```python
from build123d import *

# Parameters (mm, degrees)
F2_R      = 40
F2_R_2    = 23
F4_DEPTH  = 34
F8_DEPTH  = 25
F10_DEPTH = 34


with BuildPart() as f4:
    # F2 (on face) → F4 (new body)
    with BuildSketch(Plane(origin=(0, 0, 0), x_dir=(-1, 0, 0), z_dir=(0, 0.906308, 0.422618))):
        Circle(F2_R)
        Circle(F2_R_2, mode=Mode.SUBTRACT)
    extrude(amount=-F4_DEPTH)



with BuildPart() as f8:
    # F7 (on offset) → F8 (new body)
    with BuildSketch(Plane.YZ.offset(-46)):
        Polygon((-14.199466, -50), (-33.909734, -50), (-33.909734, -65), (-13.909734, -65), (-13.909734, -50.621332), align=None)
        Polygon((-13.909734, -50.621332), (-13.909734, -65), (-7.204851, -65), align=None)
        Polygon((23.315383, -50), (-14.199466, -50), (-13.909734, -50.621332), (-7.204851, -65), (30.309998, -65), align=None)
        Polygon((46.090266, -50), (23.315383, -50), (30.309998, -65), (46.090266, -65), align=None)
    extrude(amount=F8_DEPTH)


with BuildPart() as f4_1:
    add(f4.part)

    add(f8.part)  # F10 merges F8
    # F9 (on face) → F10 (join, through all)
    with BuildSketch(Plane(origin=(0, 0, 0), x_dir=(-1, 0, 0), z_dir=(0, 0.906308, 0.422618))):
        with BuildLine():
            Line((40, -85.627586), (40, 0))
            ThreePointArc((40, 0), (35.496479, -18.439089), (23, -32.726136))
            Line((23, -32.726136), (23, -85.627586))
            Line((23, -85.627586), (40, -85.627586))
        make_face()
    extrude(amount=-F10_DEPTH)


solid = f4_1.part
```
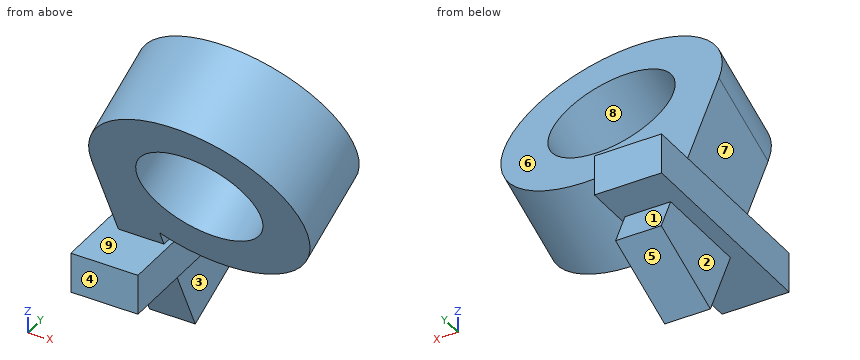
CAD build for the part. Positions are in the model's coordinates, mm. Face numbers are marked on the shaded views. A direction names the side the tool comes from. Round coordinates to 2 decimals unless told otherwise and drop trailing zeros. Write each loop counter-clockwise with the first axis right and the second up, starting at its lowest first coordinate (ties: lowest second). Pieces come first, ordered by that corner, then holes.
Item 1: Drill centre lines: L1, parallel to Z at x = -22.5, y = 5; L2, parallel to Z at x = 0, y = -16; L3, parallel to X at y = -2.5, z = -65.5. Where is each one in solid material? Low to high.
Filled in:
L1: z = -65 to -50, -34.16 to -10.72
L2: z = -46.14 to -32.84, 17.92 to 34.31
L3: x = -40 to -23
Item 2: Band-saw the part on D-D on x = -25.5. Write the cut outline in (y, z), then the cut area to 3 significant figures.
Filled in:
outline: (-43.84, 13.56) - (-14.2, -50) - (-33.91, -50) - (-33.91, -65) - (-7.2, -65) - (5.37, -91.97) - (36.19, -77.6) - (30.31, -65) - (46.09, -65) - (46.09, -50) - (23.32, -50) - (-13.02, 27.93) - close
area: 4,600 mm2
Item 3: Band-saw the part on C-C on y = 39.5. Write the cut outline in (x, z).
Filled in:
outline: (-46, -65) - (-21, -65) - (-21, -50) - (-46, -50) - close
Item 4: Tool access for the marked faces 1, 2, 3, 4 and 5: list every direction of +Z, -Z, +X, -X, +Y, -Y with a clear straight run to the whole face (end or side of a thin tool).
Filled in:
face 1: +X, -X, +Y
face 2: -Z, -X, +Y, -Y
face 3: -Z, +X, +Y, -Y
face 4: -Z, +X, -X, -Y
face 5: -Z, +X, -X, +Y
Item 5: Mould opens along Z. For the marked faces 6, 7, 8 and 9 say: released by +Z, released by -Z, zero draft, split by the parting line, or undercut.
Filled in:
face 6: released by +Z
face 7: zero draft
face 8: undercut
face 9: undercut
Item 6: Drop flat-ended pins along their axis: pin 1 Ø12 at (y, z) = (-23.5, -76) entering from +X; pin 2 Ø10 at (y, z) = (0.5, -39.5) entering from +X; pin 3 Ø20 at (x, y) = (-39.5, 23.5) entering from +Z; pin 4 Ø4.5 at (x, z) = (-34.5, -54) entering from -Y. Give the stop position or say it passes through.
Filled in:
pin 1: passes through
pin 2: stops at x = 25.27
pin 3: stops at z = -28.95
pin 4: stops at y = -33.91
Item 7: Band-saw the part on B-B on z = -62. Write the cut outline in (x, y).
Filled in:
outline: (-46, -33.91) - (-21, -33.91) - (-21, 46.09) - (-46, 46.09) - close
Item 8: Band-saw the part on A-A on x = 14. Write the cut outline in (y, z), then the cut area to 3 significant figures.
Filled in:
outline: (-46.65, 19.59) - (-38.53, 2.17) - (-7.71, 16.54) - (-15.84, 33.96) - close; (-23.1, -30.91) - (-14.98, -48.33) - (15.84, -33.96) - (7.71, -16.54) - close
area: 1,310 mm2
